Part print with two shaded views. Sizes in mm from the minimum x, y, z corner. Coordinates: 2 decimals unless noted, no trailing zeros. Order: outer loops, then holes, each group sorted by start corner. A loop starts at its lowest first (then second) coordinate and runs counter-clockwise, first axis right, second up.
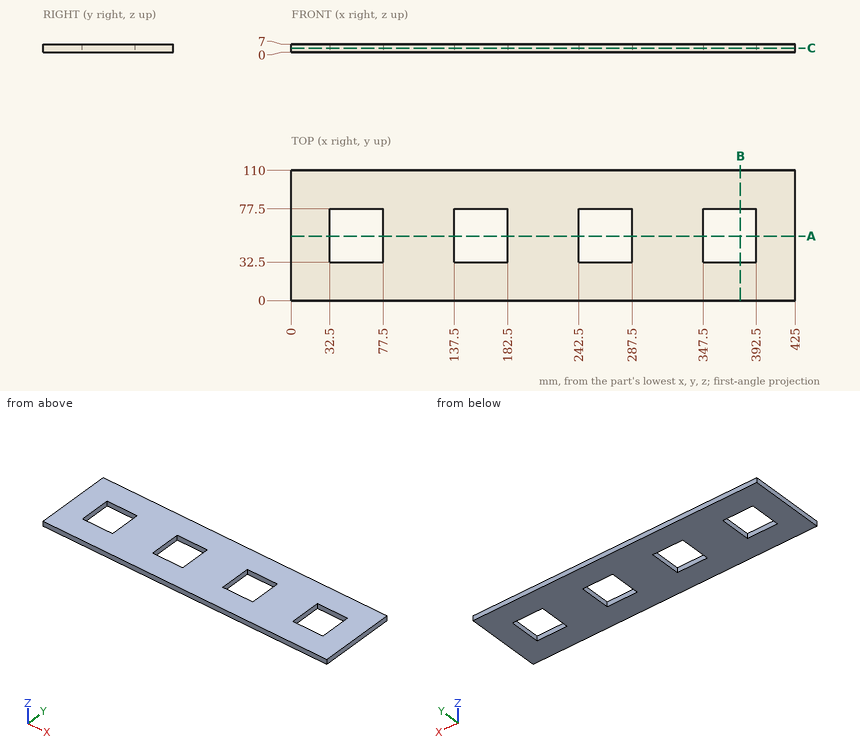
Q1. Cut at C-C on z = 3.5. Write the cut outline in (x, y).
Results list:
outline: (0, 0) - (425, 0) - (425, 110) - (0, 110) - close; hole (32.5, 32.5) - (77.5, 32.5) - (77.5, 77.5) - (32.5, 77.5) - close; hole (137.5, 32.5) - (182.5, 32.5) - (182.5, 77.5) - (137.5, 77.5) - close; hole (242.5, 32.5) - (287.5, 32.5) - (287.5, 77.5) - (242.5, 77.5) - close; hole (347.5, 32.5) - (392.5, 32.5) - (392.5, 77.5) - (347.5, 77.5) - close
Q2. Pin check, flat tip, straight feed: pin 1 Ø8 at (x, y) = (177.5, 42.5) entering from +Z. Stop position of the tip, or through.
Results list:
pin 1: passes through
Q3. Wall check: line 1 along X through (y, z) = (57, 1.25); line 2 along Y through (x, z) = (35, 1). Give the ranges that are in metal, low to high.
Results list:
line 1: x = 0 to 32.5, 77.5 to 137.5, 182.5 to 242.5, 287.5 to 347.5, 392.5 to 425
line 2: y = 0 to 32.5, 77.5 to 110
Q4. Cut at A-A on y = 54.5. Write the cut outline in (x, z), and give its area (4 significant figures).
Results list:
outline: (0, 0) - (32.5, 0) - (32.5, 7) - (0, 7) - close; (77.5, 0) - (137.5, 0) - (137.5, 7) - (77.5, 7) - close; (182.5, 0) - (242.5, 0) - (242.5, 7) - (182.5, 7) - close; (287.5, 0) - (347.5, 0) - (347.5, 7) - (287.5, 7) - close; (392.5, 0) - (425, 0) - (425, 7) - (392.5, 7) - close
area: 1,715 mm2
Q5. Cut at B-B on x = 379. Write the cut outline in (y, z), and give its area (3 significant figures).
Results list:
outline: (0, 0) - (32.5, 0) - (32.5, 7) - (0, 7) - close; (77.5, 0) - (110, 0) - (110, 7) - (77.5, 7) - close
area: 455 mm2
